Input: part model. Units: mm. Frame: model coordinates. A direction names the side the tool comes from. Coordinates: 2 decimals unless noted, no trailing zeros. Order: outer loops, then holes, each group sorted by start corner. A loop starts at its lowest first (then second) coordinate and runs counter-clockwise, first axis right, second up. Notation, with made-up numbers: (73.5, 37.5) -> (99.5, 37.5) arc R9 ccw to (99.5, 46.5) -> close; hole circle Ø11 at (45.25, 42.5). An arc over 180 degrees is marked (long way). Use one line per item in the form item = value. Start each with the question number.
1) Draft query along X for faces 1 (the flat face through (-28.116, 1.322, 20.809)), 2 (the cylindrical face through (-20.22, -0.09, 18.55)), 3 (the flat face through (28.223, -1.5, 20.702)). Return one class per face: pulls with the +X half, pulls with the -X half, needs draft (parallel to the pull), parting line crosses it, or undercut.
2) Section query D-D on x = -25. Output: boundary loops of the cut face in (y, z) (3 decimals), then the cut area to 3 significant figures.
3) Section query A-A on z = 2.25. Output: boundary loops of the cut face in (x, y) (3 decimals), then the cut area to 3 significant figures.
4) Section query C-C on x = 0. Output: boundary loops of the cut face in (y, z), then the cut area to 3 significant figures.
5) Section query B-B on y = 0. Count the separate pieces of the cut face and the enclosed holes in it, then the cut area to 3 significant figures.
6) Pin query (flat end, axial travel): pin 1 (3 mm diameter, centred on x = -20.5, y = -3.5, fed in from -Z); pin 2 (4 mm diameter, centred on x = 4.5, y = 3.5, fed in from -Z); pin 3 (4 mm diameter, centred on x = 0, y = -3, fed in from -Z); pin 4 (1 mm diameter, centred on y = 2, z = 19.5, fed in from +X) (3 decimals). Return the tip coordinate at first contact, or that it passes through.
7) Ray query, line 1 along Y through (x, z) = (0, 20.1); line 2 along X through (y, z) = (1.75, 7) (3 decimals); line 3 along Z through (x, y) = (-15.5, 4.5). Return the intervals inside material, ascending.
8) Access query for faces 4 (the cylindrical face through (-1.18, 2.26, 24.39)), 5 (the cylindrical face through (-1.19, 5.37, 19.89)), 6 (the flat face through (21.125, 0, 8)). Directions: +Z, -Z, +X, -X, +Y, -Y. A direction counts if a zero-diameter tool reaches every point of the face in a straight line with its end or side. Return the directions, or none.
from build123d import *

# Parameters (mm, degrees)
F1_DEPTH        = 6.35
F4_D            = 4.2
F6_DEPTH        = 12.701
F8_DEPTH        = 12.701
F2_R            = 5.5
F9_DEPTH        = 1
F11_D           = 5.1
F11_CSINK_D     = 11
F11_CSINK_ANGLE = 90


with BuildPart() as f1:
    # F0 (on Front) → F1 (new body, symmetric)
    with BuildSketch(Plane.XZ):
        Polygon((-31.125, 17.8), (-31.125, 0), (-21.125, 0), (-21.125, 11.8), (-13.525, 19.4), (13.525, 19.4), (21.125, 11.8), (21.125, 0), (31.125, 0), (31.125, 17.8), (23.525, 25.4), (-23.525, 25.4), align=None)
    extrude(amount=F1_DEPTH, both=True)

    # F4 (through all)
    with Locations(Plane(origin=(0, 0, 0), x_dir=(1, 0, 0), z_dir=(0, 0, -1))):
        with Locations((-26.125, 0), (26.125, 0)):
            Hole(F4_D / 2)

    # F5 (on face) → F6 (cut, through all)
    with BuildSketch(Plane.XZ.offset(6.35)):
        with BuildLine():
            ThreePointArc((-14.6379942315, 18.2870057685), (-15.870802957, 19.1107422235), (-17.325, 19.4))
            ThreePointArc((-17.325, 19.4), (-20.0120057685, 18.2870057685), (-21.125, 15.6))
            ThreePointArc((-21.125, 15.6), (-20.8357422235, 14.145802957), (-20.0120057685, 12.9129942315))
            Line((-20.0120057685, 12.9129942315), (-14.6379942315, 18.2870057685))
        make_face()
        with BuildLine():
            Line((-13.525, 19.4), (-17.325, 19.4))
            ThreePointArc((-17.325, 19.4), (-15.870802957, 19.1107422235), (-14.6379942315, 18.2870057685))
            Line((-14.6379942315, 18.2870057685), (-13.525, 19.4))
        make_face()
        with BuildLine():
            ThreePointArc((-20.0120057685, 12.9129942315), (-20.8357422235, 14.145802957), (-21.125, 15.6))
            Line((-21.125, 15.6), (-21.125, 11.8))
            Line((-21.125, 11.8), (-20.0120057685, 12.9129942315))
        make_face()
        with BuildLine():
            ThreePointArc((21.125, 15.6), (20.0120057685, 18.2870057685), (17.325, 19.4))
            ThreePointArc((17.325, 19.4), (15.870802957, 19.1107422235), (14.6379942315, 18.2870057685))
            Line((14.6379942315, 18.2870057685), (20.0120057685, 12.9129942315))
            ThreePointArc((20.0120057685, 12.9129942315), (20.8357422235, 14.145802957), (21.125, 15.6))
        make_face()
        with BuildLine():
            Line((17.325, 19.4), (13.525, 19.4))
            Line((13.525, 19.4), (14.6379942315, 18.2870057685))
            ThreePointArc((14.6379942315, 18.2870057685), (15.870802957, 19.1107422235), (17.325, 19.4))
        make_face()
        with BuildLine():
            Line((21.125, 11.8), (21.125, 15.6))
            ThreePointArc((21.125, 15.6), (20.8357422235, 14.145802957), (20.0120057685, 12.9129942315))
            Line((20.0120057685, 12.9129942315), (21.125, 11.8))
        make_face()
    extrude(amount=-F6_DEPTH, mode=Mode.SUBTRACT)

    # F7 (on face) → F8 (cut, through all)
    with BuildSketch(Plane.XZ.offset(6.35)):
        with BuildLine():
            ThreePointArc((-21.1013054614, 16.0236945386), (-20.0120057685, 18.2870057685), (-17.7486945386, 19.3763054614))
            ThreePointArc((-17.7486945386, 19.3763054614), (-20.2463203436, 18.5213203436), (-21.1013054614, 16.0236945386))
        make_face()
        with BuildLine():
            ThreePointArc((21.125, 16.4), (20.1088200039, 18.6504351117), (17.7486945386, 19.3763054614))
            ThreePointArc((17.7486945386, 19.3763054614), (20.0120057685, 18.2870057685), (21.1013054614, 16.0236945386))
            ThreePointArc((21.1013054614, 16.0236945386), (21.1190705055, 16.2114746493), (21.125, 16.4))
        make_face()
    extrude(amount=-F8_DEPTH, mode=Mode.SUBTRACT)

    # F2 (on face) → F9 (cut)
    with BuildSketch(Plane(origin=(0, 0, 19.4), x_dir=(1, 0, 0), z_dir=(0, 0, -1))):
        Circle(F2_R)
    extrude(amount=-F9_DEPTH, mode=Mode.SUBTRACT)

    # F11 (through all)
    with Locations(Plane(origin=(0, 0, 20.4), x_dir=(1, 0, 0), z_dir=(0, 0, -1))):
        with Locations((0, 0)):
            CounterSinkHole(F11_D / 2, F11_CSINK_D / 2, counter_sink_angle=F11_CSINK_ANGLE)


solid = f1.part
Answers below:
q1.face_1 = pulls with the -X half
q1.face_2 = undercut
q1.face_3 = pulls with the +X half
q2.outline = (-6.35, 0) -> (-1.773, 0) -> (-1.773, 23.925) -> (-6.35, 23.925) -> close; (1.773, 0) -> (6.35, 0) -> (6.35, 23.925) -> (1.773, 23.925) -> close
q2.area = 219 mm^2
q3.outline = (-31.125, -6.35) -> (-21.125, -6.35) -> (-21.125, 6.35) -> (-31.125, 6.35) -> close; (21.125, -6.35) -> (31.125, -6.35) -> (31.125, 6.35) -> (21.125, 6.35) -> close; hole circle Ø4.2 at (-26.125, 0); hole circle Ø4.2 at (26.125, 0)
q3.area = 226 mm^2
q4.outline = (-6.35, 19.4) -> (-5.5, 19.4) -> (-5.5, 20.4) -> (-2.55, 23.35) -> (-2.55, 25.4) -> (-6.35, 25.4) -> close; (2.55, 23.35) -> (5.5, 20.4) -> (5.5, 19.4) -> (6.35, 19.4) -> (6.35, 25.4) -> (2.55, 25.4) -> close
q4.area = 31.0 mm^2
q5.separate_pieces = 4
q5.enclosed_holes = 0
q5.area = 471 mm^2
q6.pin_1 = 0
q6.pin_2 = 19.4
q6.pin_3 = 20.9
q6.pin_4 = 29.925
q7.line_1 = -6.35 to -5.5, 5.5 to 6.35
q7.line_2 = -31.125 to -27.286, -24.964 to -21.125, 21.125 to 24.964, 27.286 to 31.125
q7.line_3 = 19.4 to 25.4
q8.face_4 = +Z, -Z
q8.face_5 = -Z
q8.face_6 = -Z, +Y, -Y
